Geometry: see drawing. Coordinates: mm, zero at the bounding-box minimum. A direction names the side the tool comes from. Round coordinates to 2 decimals unless told otherwise and drop trailing zeros. Loops run counter-clockwise (first coordinate to the right, second up) from the corner with the lowest first, then second, coordinate; pieces in that order, holes last. Notation, with made-up numbers: (-13, 86) -> (46, 86) arc R28 cw to (46, 106) -> close; hole circle Ø9 at (36.25, -8.5). An arc over 180 degrees is marked (long way). Answer in a Markdown table with one row per item.
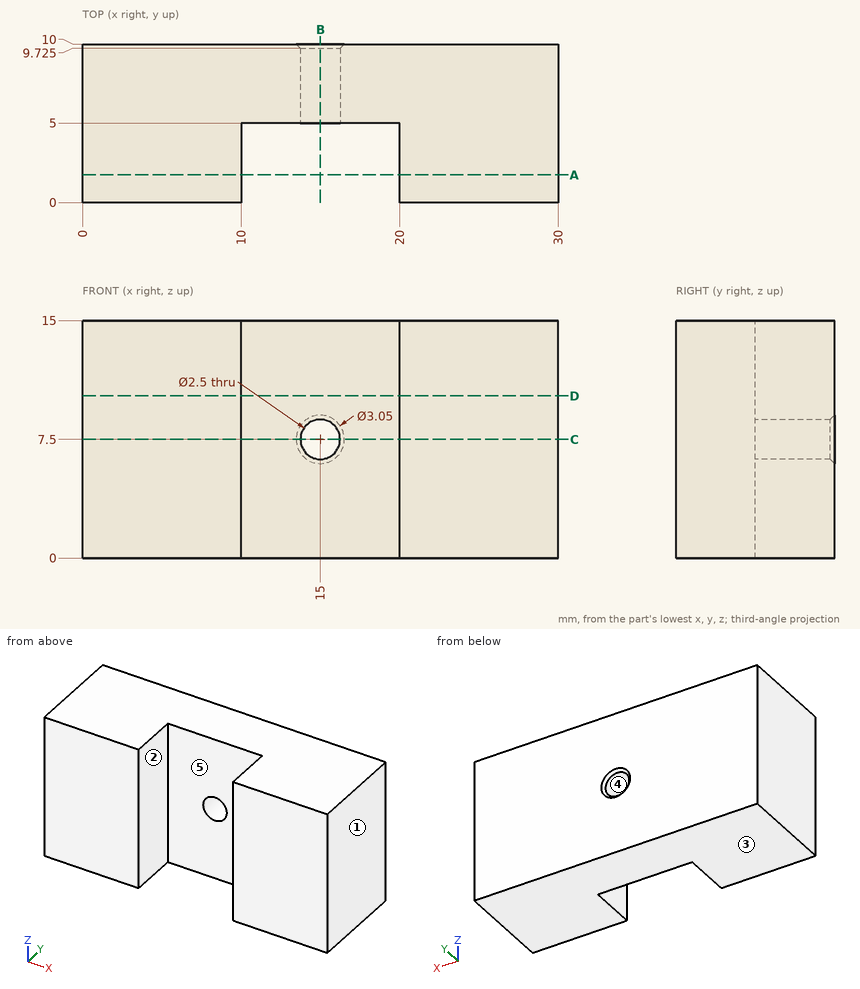
Item 1: Mould query, pull axis X, two halves, no side actions, for the marked faces 1, 2 and 3. Classes: released by +X, released by -X, zero draft, split by the parting line, or undercut.
Ans:
| item | result |
|---|---|
| face 1 | released by +X |
| face 2 | undercut |
| face 3 | zero draft |
Item 2: Set-up query: the marked faces 4 and 5. Return all of +Z, -Z, +X, -X, +Y, -Y with unobstructed straight access to the full face (end or side cutting, diameter ignored); none if empty.
Ans:
| item | result |
|---|---|
| face 4 | +Y, -Y |
| face 5 | +Z, -Z, -Y |
Item 3: First-contact query: P1, Ø4, axis at x = 23.5, z = 11.5, coming from the -Y side; P2, Ø8, axis at x = 15, z = 4, coming from the -Y side; P3, Ø1.5, axis at x = 15, z = 7.5, coming from the +Y side. Flat tips, straight axial feed; report the tip coordinate or a pass-through.
Ans:
| item | result |
|---|---|
| P1 | y = 0 |
| P2 | y = 5 |
| P3 | through |
Item 4: Section query A-A, the plane y = 1.75. Output: boundary loops of the cut face in (x, z), and give its area (3 significant figures).
Ans:
| item | result |
|---|---|
| outline | (0, 0) -> (10, 0) -> (10, 15) -> (0, 15) -> close; (20, 0) -> (30, 0) -> (30, 15) -> (20, 15) -> close |
| area | 300 mm2 |
Item 5: Ray query, L1, parallel to X at y = 3, z = 10.75; L2, parallel to X at y = 7.05, z = 7.5; L3, parallel to Z at x = 15, y = 8.1. Return the intervals inside material, ascending.
Ans:
| item | result |
|---|---|
| L1 | 0 to 10, 20 to 30 |
| L2 | 0 to 13.75, 16.25 to 30 |
| L3 | 0 to 6.25, 8.75 to 15 |
Item 6: Section query C-C, the plane z = 7.5. Output: boundary loops of the cut face in (x, y) (3 decimals).
Ans:
| item | result |
|---|---|
| outline | (0, 0) -> (10, 0) -> (10, 5) -> (13.75, 5) -> (13.75, 9.725) -> (13.475, 10) -> (0, 10) -> close; (16.25, 5) -> (20, 5) -> (20, 0) -> (30, 0) -> (30, 10) -> (16.525, 10) -> (16.25, 9.725) -> close |
Item 7: Section query B-B, the plane x = 15. Output: boundary loops of the cut face in (y, z) (3 decimals), and give its area (3 significant figures).
Ans:
| item | result |
|---|---|
| outline | (5, 0) -> (10, 0) -> (10, 5.975) -> (9.725, 6.25) -> (5, 6.25) -> close; (5, 8.75) -> (9.725, 8.75) -> (10, 9.025) -> (10, 15) -> (5, 15) -> close |
| area | 62.4 mm2 |
Item 8: Section query D-D, the plane z = 10.25. Output: boundary loops of the cut face in (x, y), and give its area (3 significant figures).
Ans:
| item | result |
|---|---|
| outline | (0, 0) -> (10, 0) -> (10, 5) -> (20, 5) -> (20, 0) -> (30, 0) -> (30, 10) -> (0, 10) -> close |
| area | 250 mm2 |
